from build123d import *

# Parameters (mm, degrees)
BOSS_EXTRUDE2_DEPTH = 14.63


with BuildPart() as part:
    # Sketch1 → Boss-Extrude2 (new body)
    with BuildSketch(Plane.XY):
        Polygon((0, 0), (-400, 0), (-800, 300), (400, 300), align=None)
        Polygon((-585.37, 157.315), (-756.11, 285.37), (-207.315, 285.37), (-207.315, 157.315), (-575.616666667, 157.315), align=None, mode=Mode.SUBTRACT)
        Polygon((-565.863333333, 142.685), (-207.315, 142.685), (-207.315, 14.63), (-395.123333333, 14.63), align=None, mode=Mode.SUBTRACT)
        Polygon((356.11, 285.37), (185.37, 157.315), (175.161951027, 157.315), (-192.685, 157.315), (-192.685, 285.37), align=None, mode=Mode.SUBTRACT)
        Polygon((-4.876666667, 14.63), (-192.685, 14.63), (-192.685, 142.685), (165.863333333, 142.685), align=None, mode=Mode.SUBTRACT)
    extrude(amount=BOSS_EXTRUDE2_DEPTH)


solid = part.part
Here's how the part is built. I have some questions about the finished solid (model axes, mm). A direction names the side the tool comes from. Give positions to 0.01 mm unless a question says otherwise; leave off trailing zeros. Order: outer loops, then holes, each group sorted by start corner. A loop starts at its lowest first (then second) coordinate and runs counter-clockwise, first axis right, second up. Notation, with made-up numbers: (-27.5, -26) -> (1.5, -26) arc R29 ccw to (1.5, 4) -> close; hole circle Ø9 at (-19, 8.25). An arc over 180 degrees is marked (long way). Use a Markdown table: item, result. Add a question column.
Item 1: I need wall thicknesses on line 1 (Y direction, x = -100, z = 4) (3 decimals); line 2 (X direction, y = 223, z = 2) (3 decimals); line 3 (X direction, y = 285, z = 8) (3 decimals). Which ranges of each line are inside material? Lowest first, please.
Item 2: If we mould it in two halves opening along X, with no side actions, what happens to faces 3 (the face through (202.8, 152.1, 7.2)), 4 (the face through (-479.298, 77.761, 7.213)), 5 (the face through (-242, 151, 14.63)), 6 (the face through (271.94, 222.24, 7.21))? For each: pulls with the +X half, pulls with the -X half, needs draft (parallel to the pull), parting line crosses it, or undercut.
Item 3: For faces 1 (the face through (-242, 151, 0)), 2 (the face through (81.689, 79.554, 7.213)), which set-ups out of +Z, -Z, +X, -X, +Y, -Y let a thin tool reach every point of the face, with its end or its side?
Item 4: Imagine slicing it at A-A on z = 5. Please give me the cut outline in (x, y) (3 decimals).
Item 5: Imagine slicing it at C-C on y = 48. Please give me the cut outline in (x, z) (3 decimals), plus the area to 3 significant figures.
Item 6: Imagine slicing it at B-B on x = -276. Please give me the cut outline in (y, z) (3 decimals), plus the area to 3 significant figures.
Item 7: Will these pins go through, and if not, where does the flat tip stop? pin 1 (7.5 mm diameter, centred on y = 62.5, z = 9, fed in from -X); pin 2 (1.5 mm diameter, centred on y = 97.5, z = 10, fed in from +X).
Data:
| question | item | result |
|---|---|---|
| 1 | line 1 | y = 0 to 14.63, 142.685 to 157.315, 285.37 to 300 |
| 1 | line 2 | x = -697.333 to -672.95, -207.315 to -192.685, 272.95 to 297.333 |
| 1 | line 3 | x = -780 to -755.617, -207.315 to -192.685, 355.617 to 380 |
| 2 | face 3 | pulls with the +X half |
| 2 | face 4 | undercut |
| 2 | face 5 | needs draft |
| 2 | face 6 | undercut |
| 3 | face 1 | -Z, +X, -X, +Y, -Y |
| 3 | face 2 | +Z, -Z |
| 4 | outline | (-800, 300) -> (-400, 0) -> (0, 0) -> (400, 300) -> close; hole (-756.11, 285.37) -> (-585.37, 157.315) -> (-207.315, 157.315) -> (-207.315, 285.37) -> close; hole (-565.863, 142.685) -> (-395.123, 14.63) -> (-207.315, 14.63) -> (-207.315, 142.685) -> close; hole (-192.685, 14.63) -> (-4.877, 14.63) -> (165.863, 142.685) -> (-192.685, 142.685) -> close; hole (-192.685, 157.315) -> (185.37, 157.315) -> (356.11, 285.37) -> (-192.685, 285.37) -> close |
| 5 | outline | (-464, 0) -> (-439.617, 0) -> (-439.617, 14.63) -> (-464, 14.63) -> close; (-207.315, 0) -> (-192.685, 0) -> (-192.685, 14.63) -> (-207.315, 14.63) -> close; (39.617, 0) -> (64, 0) -> (64, 14.63) -> (39.617, 14.63) -> close |
| 5 | area | 927 mm² |
| 6 | outline | (0, 0) -> (14.63, 0) -> (14.63, 14.63) -> (0, 14.63) -> close; (142.685, 0) -> (157.315, 0) -> (157.315, 14.63) -> (142.685, 14.63) -> close; (285.37, 0) -> (300, 0) -> (300, 14.63) -> (285.37, 14.63) -> close |
| 6 | area | 642 mm² |
| 7 | pin 1 | stops at x = -488.33 |
| 7 | pin 2 | stops at x = 131 |
